from build123d import *

# Parameters (mm, degrees)
CHAMFER_SIZE = 0.5


with BuildPart() as part:
    # Sketch → Revolution (revolve)
    with BuildSketch(Plane.YZ):
        Polygon((0, 0), (20, 0), (26, 50), (28, 50), (28.1, 60), (25.185651, 60), (18.225651, 2), (0, 2), align=None)
    revolve(axis=Axis((0, 0, 0), (0, 0, 1)))

    # Chamfer
    chamfer_edges = [part.edges().sort_by_distance(p)[0] for p in [
        (0, -20, 0),
        (0, -28, 50),
        (0, -26, 50),
        (0, -28.1, 60),
        (0, -25.185651, 60),
        (0, -18.225651, 2),
    ]]
    chamfer(chamfer_edges, length=CHAMFER_SIZE)


solid = part.part
Model file for the job. Use its own axes, mm. A direction names the side the tool comes from. Coordinates: 2 decimals unless noted, no trailing zeros. Loops run counter-clockwise (first coordinate to the right, second up) from the corner with the lowest first, then second, coordinate; pieces in that order, holes last. Notation, with made-up numbers: (56.5, -30) -> (100.5, -30) arc R10 ccw to (100.5, -17) -> close; hole circle Ø4 at (-38, -2). An arc over 180 degrees is marked (long way). Use one line per item in the form item = value. Start each with the question number.
(1) Probe probe 1 along Y at (x, z) = (-22.5, 54.5); probe 2 along Z at (x, y) = (10, -6); probe 3 along X at (y, z) = (16, 27). List the from-to ranges inside material, lowest first. Write a range as from..to.
(2) Cut at B-B on z = 25. Give the cut face in (x, y).
(3) Tool access for faces 1 (the conical face through (-8.426, 26.755, 55.063)), 2 (the flat face through (18.3, 18.3, 60)), 3 (the flat face through (0, 0, 2)): list every direction of +Z, -Z, +X, -X, +Y, -Y with a clear straight run to the whole face (end or side of a thin tool).
(4) Pull direction X, two halves, no side cores. Call faces 4 (the conical face through (13.62, -17.77, 19.9)), 5 (the flat face through (0, 0, 0)), 6 (the conical face through (-6.505, 20.658, 30.601)): pulls with the +X half, pulls with the -X half, needs draft (parallel to the pull), parting line crosses it, or undercut.
(5) Cut at A-A on z = 4.5. Give the cut face in (x, y).
(6) Flat gauge pins, fed straight in: pin 1 (8 mm diameter, centred on x = -4, z = 53, fed in from +Y); pin 2 (10 mm diameter, centred on x = 18.5, z = 22, fed in from -Y); pin 3 (3 mm diameter, centred on x = 17.5, y = -9.5, fed in from -Z); pin 4 (12 mm diameter, centred on x = -11, z = 37, fed in from -Y). Where does each tip first touch, or does it go through?
Values:
q1.probe_1 = -16.74..-9.76, 9.76..16.74
q1.probe_2 = 0..2
q1.probe_3 = -16.86..-13.95, 13.95..16.86
q2.outline = circle Ø46 at (0, 0); hole circle Ø41.97 at (0, 0)
q3.face_1 = -Z
q3.face_2 = +Z, +X, -X, +Y, -Y
q3.face_3 = +Z
q4.face_4 = parting line crosses it
q4.face_5 = needs draft
q4.face_6 = undercut
q5.outline = circle Ø41.08 at (0, 0); hole circle Ø37.05 at (0, 0)
q6.pin_1 = 28.04
q6.pin_2 = -18.25
q6.pin_3 = 0
q6.pin_4 = -24.11
